CAD build for the part. Positions are in the model's coordinates, mm. A direction names the side the tool comes from. Give positions to 0.01 mm unless a question says otherwise; leave off trailing zeros. Order: outer loops, then holes, each group sorted by start corner. A loop starts at its lowest first (then second) coordinate and runs counter-clockwise, first axis right, second up.
Autodesk Inventor part; units mm, degrees
ref_plane "YZ Plane" through (0, 0, 0) normal (1, 0, 0) x (0, 1, 0)
ref_plane "XZ Plane" through (0, 0, 0) normal (0, 1, 0) x (-1, 0, 0)
ref_plane "XY Plane" through (0, 0, 0) normal (0, 0, 1) x (1, 0, 0)
sketch "Sketch1" plane through (0, 0, 0) normal (1, 0, 0) x (0, 1, 0)
  arc A0 (13.4228, -41.8269) -> (6.5772, -34.1731) centre (10, -38) ccw
  arc A1 (-13.4228, -41.8269) -> (13.4228, -41.8269) centre (0, -26.8197) ccw
  arc A2 (-6.5772, -34.1731) -> (-13.4228, -41.8269) centre (-10, -38) ccw
  arc A3 (-6.5772, -34.1731) -> (6.5772, -34.1731) centre (0, -26.8197) ccw
  arc A4 (-41.8269, -13.4228) -> (-34.1731, -6.5772) centre (-38, -10) ccw
  arc A5 (-41.8269, 13.4228) -> (-41.8269, -13.4228) centre (-26.8197, 0) ccw
  arc A6 (-34.1731, 6.5772) -> (-41.8269, 13.4228) centre (-38, 10) ccw
  arc A7 (-34.1731, 6.5772) -> (-34.1731, -6.5772) centre (-26.8197, 0) ccw
  arc A8 (-13.4228, 41.8269) -> (-6.5772, 34.1731) centre (-10, 38) ccw
  arc A9 (13.4228, 41.8269) -> (-13.4228, 41.8269) centre (0, 26.8197) ccw
  arc A10 (6.5772, 34.1731) -> (13.4228, 41.8269) centre (10, 38) ccw
  arc A11 (6.5772, 34.1731) -> (-6.5772, 34.1731) centre (0, 26.8197) ccw
  circle A12 centre (0, 0) radius 21.5
  circle A13 centre (-35.3988, 27.25) radius 3.5
  circle A14 centre (-35.3988, -27.25) radius 3.5
  arc A15 (20.2079, 50.6151) -> (20.2079, -50.6151) centre (0, 0) ccw
  line L0 (26.5, -41.328) -> (26.5, 41.328)
  arc A16 (26.5, 41.328) -> (20.2079, 50.6151) centre (16.5, 41.328) ccw
  arc A17 (20.2079, -50.6151) -> (26.5, -41.328) centre (16.5, -41.328) ccw
  point P0 (26.5, -47.6235)
  point P1 (26.5, 47.6235)
  dimension "d4" = 10
  dimension "d5" = 10
extrude "Extrusion1" add sketch "Sketch1" along normal blind 10
sketch "Sketch2" plane through (10, 0, 0) normal (1, 0, 0) x (0, 0, -1)
  line L0 (41.328, 26.5) -> (-41.328, 26.5)
  line L1 (0, 24.5) -> (41.328, 24.5)
  line L2 (41.328, 24.5) -> (41.328, 26.5)
  line L3 (0, 24.5) -> (-41.328, 24.5)
  line L4 (-41.328, 24.5) -> (-41.328, 26.5)
  point P0 (0, 0)
extrude "Extrusion2" cut sketch "Sketch2" against normal blind 10
sketch "Sketch3" plane through (10, 0, 0) normal (1, 0, 0) x (0, 0, -1)
  circle A0 centre (-27.25, -35.3988) radius 3.5
  circle A1 centre (27.25, -35.3988) radius 3.5
  circle A2 centre (-27.25, -35.3988) radius 4
  circle A3 centre (27.25, -35.3988) radius 4
  point P0 (0, 0)
  dimension "d11" = 8
  dimension "d12" = 8
extrude "Extrusion3" cut sketch "Sketch3" against normal blind 10
properties part number "ballast_tengah"
1. Wall check: line 1 (Z direction, x = 8.75, y = -0.5); line 2 (Z direction, x = 2, y = 0); line 3 (Y direction, x = 6.75, z = -34). Give the ranges that are in metal, low to high.
2. Pin check, flat tips, straight feed: P1, Ø3, axis at x = 7, y = -7.5, coming from the +Z side; P2, Ø6.5, axis at y = -35.4, z = 27.25, coming from the -X side; P3, Ø1, axis at x = 4, y = 25.5, coming from the -Z side; P4, Ø1, axis at x = 6.5, y = 26, coming from the +Z side. Stop position of each tip, or through.
3. Saw through at A-A on z = 0. Give the cut face in (x, y), plus the area to 3 significant figures.
4. Saw through at D-D on x = 8.75. Give the cut face in (y, z).
5. Mould opens along Z. For faces 1 (the flat face through (0, -24, 1)), 2 (the cylindrical face through (4.93, -54.48, -1.49)), 3 (the cylindrical face through (4.93, 0.206, -46.953)), 4 (the cylindrical face through (4.93, 13.751, -34.494)) say: released by +Z, released by -Z, zero draft, split by the parting line, or undercut.
6. 3-axis set-ups, long thin cutter, end or side, ignore diameter. For faces 5 (the cylindrical face through (4.93, 24.73, 47.01)), 6 (the flat face through (5, 24.5, -1)), 7 (the cylindrical face through (4.93, -46.953, -0.206)): which of +Z, -Z, +X, -X, +Y, -Y reach the whole face in a straight line?
7. Saw through at C-C on z = -38. Give the cut face in (x, y), plus the area to 3 significant figures.
8. Saw through at B-B on y = 0. Give the cut face in (x, z), plus the area to 3 significant figures.
Reported:
1. line 1: z = -54.5 to -46.95, -36.67 to -21.49, 21.49 to 36.67, 46.95 to 54.5
1. line 2: z = -54.5 to -46.95, -36.69 to -21.5, 21.5 to 36.69, 46.95 to 54.5
1. line 3: y = -42.59 to -13.22, -6.78 to 6.78, 13.22 to 24.5
2. P1: stops at z = 54.17
2. P2: passes through
2. P3: stops at z = -46.6
2. P4: stops at z = 45.69
3. outline: (0, -54.5) - (10, -54.5) - (10, -46.95) - (0, -46.95) - close; (0, -36.69) - (10, -36.69) - (10, -21.5) - (0, -21.5) - close; (0, 21.5) - (10, 21.5) - (10, 24.5) - (0, 24.5) - close
3. area: 257 mm2
4. outline: (20.21, -50.62) arc R10 ccw to (26.5, -41.33) - (24.5, -41.33) - (24.5, 41.33) - (26.5, 41.33) arc R10 ccw to (20.21, 50.62) arc R54.5 ccw (long way) to start; hole (-41.83, -13.42) arc R5.13 ccw to (-34.17, -6.58) arc R9.87 cw to (-34.17, 6.58) arc R5.13 ccw to (-41.83, 13.42) arc R20.13 ccw to start; hole circle Ø8 at (-35.4, -27.25); hole circle Ø8 at (-35.4, 27.25); hole circle Ø43 at (0, 0); hole (-13.42, -41.83) arc R20.13 ccw to (13.42, -41.83) arc R5.13 ccw to (6.58, -34.17) arc R9.87 cw to (-6.58, -34.17) arc R5.13 ccw to start; hole (-13.42, 41.83) arc R5.13 ccw to (-6.58, 34.17) arc R9.87 cw to (6.58, 34.17) arc R5.13 ccw to (13.42, 41.83) arc R20.13 ccw to start
5. face 1: zero draft
5. face 2: split by the parting line
5. face 3: undercut
5. face 4: undercut
6. face 5: +Z, +X, -X, +Y
6. face 6: +X, -X, +Y
6. face 7: +X, -X
7. outline: (0, -39.07) - (10, -39.07) - (10, -15.13) - (0, -15.13) - close; (0, 15.13) - (10, 15.13) - (10, 24.5) - (0, 24.5) - close
7. area: 333 mm2
8. outline: (0, -54.5) - (10, -54.5) - (10, -46.95) - (0, -46.95) - close; (0, -36.69) - (10, -36.69) - (10, -21.5) - (0, -21.5) - close; (0, 21.5) - (10, 21.5) - (10, 36.69) - (0, 36.69) - close; (0, 46.95) - (10, 46.95) - (10, 54.5) - (0, 54.5) - close
8. area: 455 mm2
